```python
from build123d import *

# Parameters (mm, degrees)
F0_W         = 42.1587601304
F0_H         = 52.9734008014
F0_W_2       = 34.925
F0_H_2       = 47.625
F1_DEPTH     = 18.034
F2_DEPTH     = 2.54
F3_W         = 34.925
F3_H         = 18.034
F2_FACE_W    = 42.1587601304
F2_FACE_H    = 20.574
F4_DEPTH     = 10.32974
F5_W         = 42.1587601304
F5_H         = 52.9734008014
F6_DEPTH     = 2.54
F7_W         = 13.8736660592
F7_H         = 5.0836820155
F8_DEPTH     = 25.4
F9_W         = 6.2576979399
F9_H         = 1.2498646975
F10_DEPTH    = 0.635
F11_T1_DEPTH = 10.2510766125
F12_DEPTH    = 2.0923395641
F13_W        = 12.7831122372
F13_H        = 8.6434278637
F14_DEPTH    = 2.8529665433


# Not quite as in the source:
# - a fillet or chamfer that OpenCascade refuses, or shapes differently, is made with other operations: its cross-section is extruded or revolved along the edge and cut away or added


with BuildPart() as f1:
    # F0 (on Top) → F1 (new body)
    with BuildSketch(Plane.XY):
        Rectangle(F0_W, F0_H)
        Rectangle(F0_W_2, F0_H_2, mode=Mode.SUBTRACT)
    extrude(amount=F1_DEPTH)

    # F0 (on Top) → F2 (join)
    with BuildSketch(Plane.XY):
        Rectangle(F0_W, F0_H)
        Rectangle(F0_W_2, F0_H_2, mode=Mode.SUBTRACT)
        Rectangle(F0_W_2, F0_H_2)
    extrude(amount=-F2_DEPTH)

    # F3 (on face) + F2_face (on face) → F4 (cut)
    with BuildSketch(Plane.XZ.offset(-23.8125)):
        with Locations((0, 9.017)):
            Rectangle(F3_W, F3_H)
    with BuildSketch(Plane(origin=(0, 26.4867004007, 7.747), x_dir=(-1, 0, 0), z_dir=(0, 1, 0))):
        Rectangle(F2_FACE_W, F2_FACE_H)
    extrude(amount=-F4_DEPTH, dir=(0, -1, 0), mode=Mode.SUBTRACT)

    # F5 (on face) → F6 (join)
    with BuildSketch(Plane.XY.offset(18.034)):
        Rectangle(F5_W, F5_H)
    extrude(amount=F6_DEPTH)

    # F7 (on face) → F8 (cut)
    with BuildSketch(Plane.XZ.offset(26.4867004007)):
        with Locations((7.517300779, 13.6317610741)):
            Rectangle(F7_W, F7_H)
    extrude(amount=-F8_DEPTH, mode=Mode.SUBTRACT)

    # F9 (on face) → F10 (join)
    with BuildSketch(Plane.XY):
        with Locations((0, 25.5755782127)):
            Rectangle(F9_W, F9_H)
    extrude(amount=F10_DEPTH)

    # F11: fillet of radius 0.8197700228 on 2 edges, made by hand

    # F11_s2 → F11_t1 (cut)
    with BuildSketch(Plane.YZ.offset(-5.1255383063)):
        with BuildLine():
            ThreePointArc((26.2005105615, 0), (25.9120083094, 0.4569042778), (25.4018348269, 0.635))
            Line((25.4018348269, 0.635), (26.2005105615, 0.635))
            Line((26.2005105615, 0.635), (26.2005105615, 0))
        make_face()
        with BuildLine():
            ThreePointArc((24.950645864, 0), (25.2391481161, 0.4569042778), (25.7493215985, 0.635))
            Line((25.7493215985, 0.635), (24.950645864, 0.635))
            Line((24.950645864, 0.635), (24.950645864, 0))
        make_face()
    extrude(amount=F11_T1_DEPTH, mode=Mode.SUBTRACT)

    # F12 (add): a face of the model
    f12_faces = [f1.faces().sort_by_distance(p)[0] for p in [
        (-17.4625, 1.3371002004, 9.017),
    ]]
    extrude(f12_faces, amount=F12_DEPTH)

    # F13 (on face) → F14 (cut)
    with BuildSketch(Plane.XZ.offset(26.4867004007)):
        with Locations((-9.5031157834, 10.0388908759)):
            Rectangle(F13_W, F13_H)
    extrude(amount=-F14_DEPTH, mode=Mode.SUBTRACT)


solid = f1.part
```
Read the model definition and answer for the solid it produces. Units are mm, in the model's axes. A direction names the side the tool comes from. Give positions to 0.01 mm unless a question says otherwise; leave off trailing zeros. Write each loop counter-clockwise with the first axis right and the second up, starting at its lowest first coordinate (ties: lowest second). Pieces come first, ordered by that corner, then holes. Notation, with made-up numbers: (-30, -39) -> (2, -39) arc R28 cw to (2, -18) -> close; hole circle Ø1 at (52.5, 38). An arc over 180 degrees is marked (long way). Answer as a JSON object with one key per item and string values.
1) Section D-D on x = -2 is taken. Write down the section's boundary in (y, z), then the cut area to 3 significant figures.
Findings below:
{"outline": "(-26.49, -2.54) -> (26.49, -2.54) -> (26.49, 0) -> (26.2, 0) arc R0.82 ccw to (25.58, 0.62) arc R0.82 ccw to (24.95, 0) -> (-23.81, 0) -> (-23.81, 18.03) -> (26.49, 18.03) -> (26.49, 20.57) -> (-26.49, 20.57) -> close", "area": "318 mm^2"}
2) Section C-C on y = -15 is taken. Write down the section's boundary in (x, z), then the cut area to 3 significant figures.
Findings below:
{"outline": "(-21.08, -2.54) -> (21.08, -2.54) -> (21.08, 20.57) -> (-21.08, 20.57) -> close; hole (-15.37, 0) -> (17.46, 0) -> (17.46, 18.03) -> (-15.37, 18.03) -> close", "area": "382 mm^2"}
3) Flat-ended cylindrical pins translate along their axes: pin 1 Ø0.6 at (x, z) = (-15.5, 10) entering from -Y; pin 2 Ø3 at (x, z) = (-4.5, 6.5) entering from +Y; pin 3 Ø1 at (x, z) = (-4.5, 9) entering from +Y. Find the tip coordinate at first contact, or state that the pin passes through.
Findings below:
{"pin 1": "stops at y = -23.63", "pin 2": "stops at y = -23.81", "pin 3": "passes through"}
4) For a pull along Y with two mould halves and no side action, classify faces 1 (the flat face through (0, -26.487, 9)), 2 (the flat face through (1, 1, 0)), 3 (the flat face through (0, 26.487, 19)), 4 (the flat face through (0, 0, -2.54)) as pulls with the +Y half, pulls with the -Y half, needs draft (parallel to the pull), parting line crosses it, or undercut.
Findings below:
{"face 1": "pulls with the -Y half", "face 2": "undercut", "face 3": "pulls with the +Y half", "face 4": "needs draft"}
5) Section A-A on z = 7.25 is taken. Write down the section's boundary in (x, y), then the cut area to 3 significant figures.
Findings below:
{"outline": "(-21.08, -26.49) -> (-15.89, -26.49) -> (-15.89, -23.63) -> (-15.37, -23.63) -> (-15.37, 26.49) -> (-21.08, 26.49) -> close; (-3.11, -26.49) -> (21.08, -26.49) -> (21.08, 26.49) -> (17.46, 26.49) -> (17.46, -23.81) -> (-3.11, -23.81) -> close", "area": "548 mm^2"}
6) Straight lines are drawn through the part: probe 1 along X at (y, z) = (-24, 13.25); probe 2 along X at (y, z) = (11, 15.25); probe 3 along Z at (x, y) = (17, 4.5). For each, find the intervals that lie inside material, in ascending order. Write a range as from..to.
Findings below:
{"probe 1": "x = -21.08..-15.89, -3.11..0.58, 14.45..21.08", "probe 2": "x = -21.08..-15.37, 17.46..21.08", "probe 3": "z = -2.54..0, 18.03..20.57"}
7) A tool of negligible diameter and unlimited length cuts with its end or side. For faces 5 (the flat face through (-3.112, -25, 10)), 6 (the flat face through (-15.895, -25, 10)), 7 (the flat face through (-21.079, 0, 9)), 8 (the flat face through (0, 0, 20.574)), 9 (the flat face through (-15.37, 1, 9)), from which of +Z, -Z, +X, -X, +Y, -Y can it reach the whole face along a straight path? Write none if from no direction.
Findings below:
{"face 5": "+Y, -Y", "face 6": "-Y", "face 7": "+Z, -Z, -X, +Y, -Y", "face 8": "+Z, +X, -X, +Y, -Y", "face 9": "+Y"}
8) Section B-B on z = 11.75 is taken. Write down the section's boundary in (x, y).
Findings below:
{"outline": "(-21.08, -26.49) -> (-15.89, -26.49) -> (-15.89, -23.63) -> (-15.37, -23.63) -> (-15.37, 26.49) -> (-21.08, 26.49) -> close; (-3.11, -26.49) -> (0.58, -26.49) -> (0.58, -23.81) -> (-3.11, -23.81) -> close; (14.45, -26.49) -> (21.08, -26.49) -> (21.08, 26.49) -> (17.46, 26.49) -> (17.46, -23.81) -> (14.45, -23.81) -> close"}
